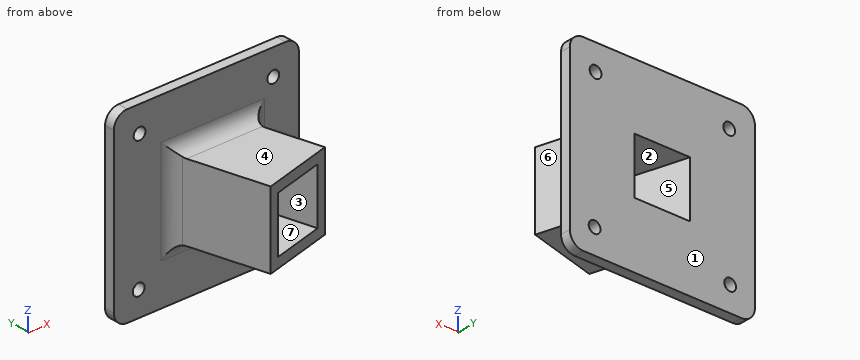
from build123d import *

# Parameters (mm, degrees)
SKETCH1_W                       = 55
SKETCH1_H                       = 55
SKETCH1_R                       = 1.75
BOSS_EXTRUDE1_DEPTH             = 3
BOSS_EXTRUDE3_REACH             = 67.033
SKETCH7_W                       = 21.733331091
SKETCH7_H                       = 22.5
SKETCH7_W_2                     = 15.937776134
SKETCH7_H_2                     = 16.5
BOSS_EXTRUDE3_DIRECTION_2_DEPTH = 11
SKETCH8_W                       = 15.937776134
SKETCH8_H                       = 16.5
CUT_EXTRUDE2_DEPTH              = 30
FILLET3_R                       = 4


with BuildPart() as part:
    # Sketch1 → Boss-Extrude1 (new body)
    with BuildSketch(Plane(origin=(0, 0, 0), x_dir=(1, 0, 0), z_dir=(0, 1, 0))):
        Rectangle(SKETCH1_W, SKETCH1_H)
        with Locations(Location((20.140368527, 20.140368527, 0), (0, 0, 270))):
            Circle(SKETCH1_R, mode=Mode.SUBTRACT)
        with Locations(Location((-19.859631473, -19.859631473, 0), (0, 0, 270))):
            Circle(SKETCH1_R, mode=Mode.SUBTRACT)
        with Locations(Location((-20.140368527, 20.140368527, 0), (0, 0, 90))):
            Circle(SKETCH1_R, mode=Mode.SUBTRACT)
        with Locations(Location((19.859631473, -19.859631473, 0), (0, 0, 90))):
            Circle(SKETCH1_R, mode=Mode.SUBTRACT)
    extrude(amount=BOSS_EXTRUDE1_DEPTH)

    # Boss-Extrude3: up to this plane
    boss_extrude3_end = Plane(origin=(0, 0, 0), z_dir=(0, 1, 0))
    # Sketch7 → Boss-Extrude3 (add, up to the surface)
    with BuildSketch(Plane(origin=(3.41851723, -12.758079989, 27.5), x_dir=(0.9659258262890681, 0.25881904510252174, 0), z_dir=(-0.25881904510252174, 0.9659258262890681, 0)), mode=Mode.PRIVATE) as boss_extrude3_sk1:
        with Locations((0.776457136, 27.5)):
            Rectangle(SKETCH7_W, SKETCH7_H)
        with Locations((0.776457135, 27.5)):
            Rectangle(SKETCH7_W_2, SKETCH7_H_2, mode=Mode.SUBTRACT)
    boss_extrude3_tool1 = split(extrude(boss_extrude3_sk1.sketch, amount=BOSS_EXTRUDE3_REACH, mode=Mode.PRIVATE), bisect_by=boss_extrude3_end, keep=Keep.BOTH, mode=Mode.PRIVATE)
    add(boss_extrude3_tool1.solids().sort_by_distance((4.168517, -12.557118, 10.937176))[0])

    # Sketch7 → Boss-Extrude3 direction 2 (add)
    with BuildSketch(Plane(origin=(3.41851723, -12.758079989, 27.5), x_dir=(0.9659258262890681, 0.25881904510252174, 0), z_dir=(-0.25881904510252174, 0.9659258262890681, 0))):
        with Locations((0.776457136, 27.5)):
            Rectangle(SKETCH7_W, SKETCH7_H)
        with Locations((0.776457135, 27.5)):
            Rectangle(SKETCH7_W_2, SKETCH7_H_2, mode=Mode.SUBTRACT)
    extrude(amount=-BOSS_EXTRUDE3_DIRECTION_2_DEPTH)

    # Sketch8 → Cut-Extrude2 (cut)
    with BuildSketch(Plane(origin=(6.265526726, -23.383264078, 0), x_dir=(0.9659258262890681, 0.2588190451025216, 0), z_dir=(0.2588190451025216, -0.9659258262890681, 0))):
        with Locations((0.776457135, 0)):
            Rectangle(SKETCH8_W, SKETCH8_H)
    extrude(amount=-CUT_EXTRUDE2_DEPTH, mode=Mode.SUBTRACT)

    # Fillet3
    fillet3_edges = [part.edges().sort_by_distance(p)[0] for p in [
        (0.803847577, 0, 11.25),
        (12.053847577, 0, 0),
        (0.803847577, 0, -11.25),
        (-10.446152423, 0, 0),
        (27.5, 1.5, 27.5),
        (-27.5, 1.5, 27.5),
        (-27.5, 1.5, -27.5),
        (27.5, 1.5, -27.5),
    ]]
    fillet(fillet3_edges, radius=FILLET3_R)


solid = part.part
Can you work these out from the model? Positions are in its coordinate system, mm. Face numbers are marked on the shaded views. A direction names the side the tool comes from. Give positions to 0.01 mm unless a question says otherwise; leave off trailing zeros. Loops run counter-clockwise (first coordinate to the right, second up) from the corner with the lowest first, then second, coordinate; pieces in that order, holes last. Notation, with made-up numbers: (4.5, 71) -> (17.5, 71) arc R30 cw to (17.5, 99) -> close; hole circle Ø5 at (44.5, -26.75). An arc over 180 degrees is marked (long way). Return JSON: item names as keys, results as strings.
Q1. I want a section at B-B, the plane x = 16.5. List the corners of the cut face in (y, z) for me, then the cut area to 3 significant figures.
Checks:
{"outline": "(-20.64, -11.25) -> (-16.59, -11.25) -> (-16.59, 11.25) -> (-20.64, 11.25) -> close; (-0.07, -14.48) arc R4 cw to (0, -15.25) -> (0, -27.5) -> (3, -27.5) -> (3, 27.5) -> (0, 27.5) -> (0, 15.25) arc R4 cw to (-0.07, 14.48) -> close", "area": "258 mm2"}
Q2. I want a section at C-C, the plane y = -18.5. List the corners of the cut face in (x, z) for me, then the cut area to 3 significant figures.
Checks:
{"outline": "(-5.49, -11.25) -> (17.01, -11.25) -> (17.01, 11.25) -> (-5.49, 11.25) -> close; hole (-2.49, -8.25) -> (14.01, -8.25) -> (14.01, 8.25) -> (-2.49, 8.25) -> close", "area": "234 mm2"}
Q3. For pin 1 Ø4 at (x, y) = (8.5, -20) entering from +Z; pin 2 Ø11.5 at (x, y) = (-1.5, -11.5) entering from -Z; pin 3 Ø3 at (x, z) = (20.14, -20.14) entering from -Y; pin 4 Ø4 at (y, z) = (-9.5, -2) entering from -X, each with a flat end and sliding along its axis, tell me the tip position at first contact or that it passes through.
Checks:
{"pin 1": "stops at z = 11.25", "pin 2": "stops at z = -11.25", "pin 3": "passes through", "pin 4": "stops at x = -8.44"}
Q4. I want a section at D-D, the plane y = 0.75. List the corners of the cut face in (x, z) for me, then the cut area to 3 significant figures.
Checks:
{"outline": "(-27.5, -23.5) arc R4 ccw to (-23.5, -27.5) -> (23.5, -27.5) arc R4 ccw to (27.5, -23.5) -> (27.5, 23.5) arc R4 ccw to (23.5, 27.5) -> (-23.5, 27.5) arc R4 ccw to (-27.5, 23.5) -> close; hole circle Ø3.5 at (-20.14, -20.14); hole circle Ø3.5 at (-19.86, 19.86); hole (-7.65, -8.25) -> (8.85, -8.25) -> (8.85, 8.25) -> (-7.65, 8.25) -> close; hole circle Ø3.5 at (19.86, 19.86); hole circle Ø3.5 at (20.14, -20.14)", "area": "2,700 mm2"}
Q5. I want a section at A-A, the plane z = 1.5. List the corners of the cut face in (x, y) for me.
Checks:
{"outline": "(-27.5, 0) -> (-13.52, 0) arc R4 cw to (-9.65, -2.96) -> (-3.48, -25.99) -> (-0.68, -25.24) -> (-8.25, 3) -> (-27.5, 3) -> close; (8.25, 3) -> (14.71, -21.12) -> (17.51, -20.37) -> (13.4, -5.04) arc R4 cw to (17.27, 0) -> (27.5, 0) -> (27.5, 3) -> close"}
Q6. I need wall thicknesses on probe 1 along Z at (x, y) = (2.5, -3); probe 2 along Z at (x, y) = (14, -19.5); probe 3 along Z at (x, y) = (-21, 1.25). Which ranges of each line are inside material? Lowest first, please.
Checks:
{"probe 1": "z = -11.38 to -8.25, 8.25 to 11.38", "probe 2": "z = -11.25 to -8.25, 8.25 to 11.25", "probe 3": "z = -27.5 to -21.66, -18.62 to 18.53, 21.19 to 27.5"}
Q7. On a 3-axis mill with a long thin cutter (end or side, diameter ignored), from which of +Z, -Z, +X, -X, +Y, -Y can I reach the whole of each face in a straight line? I mean the marked faces 1, 2 and 3. Say none if no direction works.
Checks:
{"face 1": "+Z, -Z, +X, -X, +Y", "face 2": "none", "face 3": "-Y"}
Q8. We'd pull the mould along Z, two halves only. Please class the marked faces 4, 5, 6 and 7: released by +Z, released by -Z, zero draft, split by the parting line, or undercut.
Checks:
{"face 4": "released by +Z", "face 5": "undercut", "face 6": "zero draft", "face 7": "undercut"}
